```python
from build123d import *

# Parameters (mm, degrees)
F0_R      = 26.9875
F1_DEPTH  = 17.78
F1_TAPER  = 3
F2_R      = 3.175
F3_R      = 6.35
F4_DEPTH  = 2.54
F7_DEPTH  = 12.7
F8_R      = 5.08
F9_R      = 2.54
F11_DEPTH = 15.24


# Not quite as in the source:
# - a fillet or chamfer that OpenCascade refuses, or shapes differently, is made with other operations: its cross-section is extruded or revolved along the edge and cut away or added


with BuildPart() as f1:
    # F0 (on Top) → F1 (new body)
    with BuildSketch(Plane.XY):
        Circle(F0_R)
    extrude(amount=F1_DEPTH, taper=F1_TAPER)

    # F2
    f2_edges = [f1.edges().sort_by_distance(p)[0] for p in [
        (-26.05569, 0, 17.78),
    ]]
    fillet(f2_edges, radius=F2_R)

    # F3 (on face) → F4 (cut)
    with BuildSketch(Plane.XY.offset(17.78)):
        with Locations((0, -15.24)):
            Circle(F3_R)
    extrude(amount=-F4_DEPTH, mode=Mode.SUBTRACT)

    # F5: fillet of radius 5.08 on 1 edges, made by hand

    # F5_s1 → F5_t2 (revolve)
    with BuildSketch(Plane.XZ.offset(15.24)):
        with BuildLine():
            ThreePointArc((6.35, 17.78), (4.4905909488, 15.9205909488), (1.9505909488, 15.24))
            Line((1.9505909488, 15.24), (6.35, 15.24))
            Line((6.35, 15.24), (6.35, 17.78))
        make_face()
    revolve(axis=Axis((0, -15.24, 15.24), (0, 0, 1)))

    # F6 (on face) → F7 (cut)
    with BuildSketch(Plane(origin=(0, 0, 0), x_dir=(1, 0, 0), z_dir=(0, 0, -1))):
        with BuildLine():
            ThreePointArc((1.27, 9.4399536545), (0, -9.525), (-1.27, 9.4399536545))
            Line((-1.27, 9.4399536545), (-1.27, 23.7786092161))
            ThreePointArc((-1.27, 23.7786092161), (0, -23.8125), (1.27, 23.7786092161))
            Line((1.27, 23.7786092161), (1.27, 9.4399536545))
        make_face()
    extrude(amount=-F7_DEPTH, mode=Mode.SUBTRACT)

    # F8
    f8_edges = [f1.edges().sort_by_distance(p)[0] for p in [
        (0, 23.8125, 12.7),
    ]]
    fillet(f8_edges, radius=F8_R)

    # F9
    f9_edges = [f1.edges().sort_by_distance(p)[0] for p in [
        (0, 9.525, 12.7),
    ]]
    fillet(f9_edges, radius=F9_R)

    # F10 (on face) → F11 (cut)
    with BuildSketch(Plane(origin=(0, 0, 0), x_dir=(1, 0, 0), z_dir=(0, 0, -1))):
        with BuildLine():
            Line((-2.6396454307, -1.524), (2.6396454307, -1.524))
            ThreePointArc((2.6396454307, -1.524), (0, 3.048), (-2.6396454307, -1.524))
        make_face()
    extrude(amount=-F11_DEPTH, mode=Mode.SUBTRACT)


solid = f1.part
```
Work out the finished part from the listing and answer in its coordinate system (mm). A direction names the side the tool comes from. Give positions to 0.01 mm unless a question says otherwise; leave off trailing zeros. Write each loop counter-clockwise with the first axis right and the second up, starting at its lowest first coordinate (ties: lowest second). Pieces come first, ordered by that corner, then holes. Notation, with made-up numbers: (82.25, 49) -> (117.25, 49) arc R23 ccw to (117.25, 60) -> close; hole circle Ø6 at (41, 29.5). An arc over 180 degrees is marked (long way). Write each question's results on one line, items separated by ' | '.
1. A tool of negligible diameter and unlimited length cuts with its end or side. For faces 1 (the flat face through (-0.26, 12.23, 12.7)), 2 (the flat face through (0, 0, 17.78)), 3 (the flat face through (0, -15, 15.24)), from which of +Z, -Z, +X, -X, +Y, -Y can it reach the whole face along a straight path? Write none if from no direction.
Data:
face 1: -Z | face 2: +Z, +X, -X, +Y, -Y | face 3: +Z
2. Each of these flat-tipped pins is pushed along its axis until it touches: pin 1 Ø2 at (x, y) = (-1, -15.5) entering from +Z; pin 2 Ø5 at (x, y) = (-1.5, -1) entering from -Z; pin 3 Ø1.5 at (y, z) = (6, 15) entering from -X; pin 4 Ø6.5 at (y, z) = (-16, 3.5) entering from +X. Where does it stop, or does it pass through?
Data:
pin 1: z = 15.24 | pin 2: z = 0 | pin 3: x = -25.68 | pin 4: x = 23.59
3. Find section B-B on z = 14. Determine the outline of the cut face in (x, y), and give its area (3 significant figures).
Data:
outline: circle Ø52.51 at (0, 0); hole (-2.64, 1.52) arc R3.05 ccw (long way) to (2.64, 1.52) -> close | area: 2,140 mm^2
4. Find section A-A on z = 2. Give the number of separate pieces and of enclosed holes in the cut face, and give its area (3 significant figures).
Data:
separate pieces: 1 | enclosed holes: 2 | area: 787 mm^2
5. Straight lines are drawn through the part: L1, parallel to X at y = -7.5, z = 7; L2, parallel to X at y = 0, z = 4.5 (1 decimal); L3, parallel to X at y = 0, z = 5 (1 decimal). For each, find the intervals that lie inside material, in ascending order.
Data:
L1: -25.54 to -22.6, -5.87 to 5.87, 22.6 to 25.54 | L2: -26.8 to -23.8, -9.5 to -3, 3 to 9.5, 23.8 to 26.8 | L3: -26.7 to -23.8, -9.5 to -3, 3 to 9.5, 23.8 to 26.7
6. Determine the mould class of faces 4 (the flat face through (0, -4, 0)), 5 (the flat face through (-1.27, -17, 6)), 6 (the cylindrical face through (-1.03, 23.79, 3.76)), 7 (the conical face through (-21.037, -16.13, 9.13)) for opening direction Y: +Y half, -Y half, draft (parallel to the pull), parting line (faces both ways), or undercut.
Data:
face 4: draft | face 5: undercut | face 6: undercut | face 7: parting line
